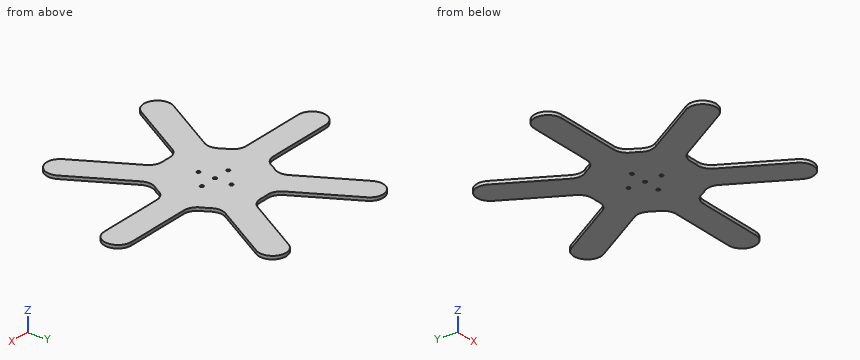
```python
from build123d import *

# Parameters (mm, degrees)
CROQUIS1_R              = 1.55
SALIENTE_EXTRUIR1_DEPTH = 1.5


with BuildPart() as part:
    # Croquis1 → Saliente-Extruir1 (new, symmetric)
    with BuildSketch(Plane.XY):
        with BuildLine():
            Line((-52.753601773, 12.7), (-114.3, 12.7))
            ThreePointArc((-114.3, 12.7), (-127, 0), (-114.3, -12.7))
            Line((-114.3, -12.7), (-52.753601773, -12.7))
            ThreePointArc((-52.753601773, -12.7), (-45.996397628, -14.646851989), (-41.310890543, -19.890520922))
            ThreePointArc((-41.310890543, -19.890520922), (-39.707264764, -22.925), (-37.881141685, -25.831020202))
            ThreePointArc((-37.881141685, -25.831020202), (-35.682744722, -32.510622834), (-37.375323514, -39.335959276))
            Line((-37.375323514, -39.335959276), (-68.148522628, -92.636703653))
            ThreePointArc((-68.148522628, -92.636703653), (-63.5, -109.985226281), (-46.151477372, -105.336703653))
            Line((-46.151477372, -105.336703653), (-15.378278258, -52.035959276))
            ThreePointArc((-15.378278258, -52.035959276), (-10.313652906, -47.157474823), (-3.429748858, -45.721541124))
            ThreePointArc((-3.429748858, -45.721541124), (0, -45.85), (3.429748858, -45.721541124))
            ThreePointArc((3.429748858, -45.721541124), (10.313652906, -47.157474823), (15.378278258, -52.035959276))
            Line((15.378278258, -52.035959276), (46.151477372, -105.336703653))
            ThreePointArc((46.151477372, -105.336703653), (63.5, -109.985226281), (68.148522628, -92.636703653))
            Line((68.148522628, -92.636703653), (37.375323514, -39.335959276))
            ThreePointArc((37.375323514, -39.335959276), (35.682744722, -32.510622834), (37.881141685, -25.831020202))
            ThreePointArc((37.881141685, -25.831020202), (39.707264764, -22.925), (41.310890543, -19.890520922))
            ThreePointArc((41.310890543, -19.890520922), (45.996397628, -14.646851989), (52.753601773, -12.7))
            Line((52.753601773, -12.7), (114.3, -12.7))
            ThreePointArc((114.3, -12.7), (127, 0), (114.3, 12.7))
            Line((114.3, 12.7), (52.753601773, 12.7))
            ThreePointArc((52.753601773, 12.7), (45.996397628, 14.646851989), (41.310890543, 19.890520922))
            ThreePointArc((41.310890543, 19.890520922), (39.707264764, 22.925), (37.881141685, 25.831020202))
            ThreePointArc((37.881141685, 25.831020202), (35.682744722, 32.510622834), (37.375323514, 39.335959276))
            Line((37.375323514, 39.335959276), (68.148522628, 92.636703653))
            ThreePointArc((68.148522628, 92.636703653), (63.5, 109.985226281), (46.151477372, 105.336703653))
            Line((46.151477372, 105.336703653), (15.378278258, 52.035959276))
            ThreePointArc((15.378278258, 52.035959276), (10.313652906, 47.157474823), (3.429748858, 45.721541124))
            ThreePointArc((3.429748858, 45.721541124), (0, 45.85), (-3.429748858, 45.721541124))
            ThreePointArc((-3.429748858, 45.721541124), (-10.313652906, 47.157474823), (-15.378278258, 52.035959276))
            Line((-15.378278258, 52.035959276), (-46.151477372, 105.336703653))
            ThreePointArc((-46.151477372, 105.336703653), (-63.5, 109.985226281), (-68.148522628, 92.636703653))
            Line((-68.148522628, 92.636703653), (-37.375323514, 39.335959276))
            ThreePointArc((-37.375323514, 39.335959276), (-35.682744722, 32.510622834), (-37.881141685, 25.831020202))
            ThreePointArc((-37.881141685, 25.831020202), (-39.707264764, 22.925), (-41.310890543, 19.890520922))
            ThreePointArc((-41.310890543, 19.890520922), (-45.996397628, 14.646851989), (-52.753601773, 12.7))
        make_face()
        Circle(CROQUIS1_R, mode=Mode.SUBTRACT)
        with Locations((0, 15.5)):
            Circle(CROQUIS1_R, mode=Mode.SUBTRACT)
        with Locations((15.5, 0)):
            Circle(CROQUIS1_R, mode=Mode.SUBTRACT)
        with Locations((0, -15.5)):
            Circle(CROQUIS1_R, mode=Mode.SUBTRACT)
        with Locations((-15.5, 0)):
            Circle(CROQUIS1_R, mode=Mode.SUBTRACT)
    extrude(amount=SALIENTE_EXTRUIR1_DEPTH, both=True)


solid = part.part
```
Work out the finished part from the listing and answer in its coordinate system (mm). Give positions to 0.01 mm unless a question says otherwise; leave off trailing zeros. Write each loop counter-clockwise with the first axis right and the second up, starting at its lowest first coordinate (ties: lowest second). Pieces come first, ordered by that corner, then holes. Notation, with made-up numbers: (84.25, 36.25) -> (99.25, 36.25) arc R22 ccw to (99.25, 43.25) -> close; hole circle Ø2 at (70, -14.75). An arc over 180 degrees is marked (long way). Write item = value, one per line.
Q1. Section C-C on z = -0.2 is taken. State how many separate pieces and enclosed holes the cut face has, and give its area (3 significant figures).
Computed values:
separate_pieces = 1
enclosed_holes = 5
area = 18,800 mm^2
Q2. Section D-D on x = 8.5 is taken. Determine the outline of the cut face in (y, z).
Computed values:
outline = (-46.37, -1.5) -> (46.37, -1.5) -> (46.37, 1.5) -> (-46.37, 1.5) -> close
Q3. Section B-B on y = -65.5 is taken. Determine the outline of the cut face in (x, z), and give its area (3 significant figures).
Computed values:
outline = (-52.48, -1.5) -> (-23.15, -1.5) -> (-23.15, 1.5) -> (-52.48, 1.5) -> close; (23.15, -1.5) -> (52.48, -1.5) -> (52.48, 1.5) -> (23.15, 1.5) -> close
area = 176 mm^2
Q4. Section A-A on x = -57.15 is taken. Determine the outline of the cut face in (y, z).
Computed values:
outline = (-111.69, -1.5) -> (-73.59, -1.5) -> (-73.59, 1.5) -> (-111.69, 1.5) -> close; (-12.7, -1.5) -> (12.7, -1.5) -> (12.7, 1.5) -> (-12.7, 1.5) -> close; (73.59, -1.5) -> (111.69, -1.5) -> (111.69, 1.5) -> (73.59, 1.5) -> close
Q5. Consider line 1 along Y through (x, z) = (0, -0.6); line 2 along Y through (x, z) = (44, -0.8); line 3 along Y through (x, z) = (-63.5, -0.8). Determine where each line is inside the solid, lowest interval first.
Computed values:
line_1 = -45.85 to -17.05, -13.95 to -1.55, 1.55 to 13.95, 17.05 to 45.85
line_2 = -101.61 to -50.81, -16.2 to 16.2, 50.81 to 101.61
line_3 = -109.99 to -84.59, -12.7 to 12.7, 84.59 to 109.99
Q6. Flat-ended cylindrical pins translate along their axes: pin 1 Ø3 at (x, y) = (-15.5, 0) entering from -Z; pin 2 Ø1.5 at (x, z) = (75, -0.5) entering from -Y; pin 3 Ø1.5 at (x, z) = (51, -1) entering from -Y; pin 4 Ø1.5 at (x, z) = (73.5, 0.5) entering from +Y. Find the tip coordinate at first contact, or state that the pin passes through.
Computed values:
pin_1 = through
pin_2 = -12.7
pin_3 = -110.48
pin_4 = 12.7
